Source: CAD feature listing. Evaluate the final solid. Frame: model axes, mm. Coordinates: 2 decimals unless noted, no trailing zeros. Order: outer loops, then holes, each group sorted by start corner. A loop starts at its lowest first (then second) coordinate and runs counter-clockwise, first axis right, second up.
Item 1: Section A-A on z = -14.5. Return the cut outline in (x, y).
Item 2: Section C-C on x = 3.35. State how many separate pieces and enclosed holes the cut face has, then the cut area to 3 significant figures.
Item 3: Ray query, line 1 (Z direction, x = 3.15, y = 330.2); line 2 (Z direction, x = 1.1, y = 429); line 3 (Y direction, x = 2, z = 17.5). Return the intervals inside material, ascending.
Item 4: Section B-B on y = 362. Return the cut outline in (x, z), then the cut area to 3 significant figures.
Autodesk Inventor part; units mm, degrees
ref_plane "YZ Plane" through (0, 0, 0) normal (1, 0, 0) x (0, 1, 0)
ref_plane "XZ Plane" through (0, 0, 0) normal (0, 1, 0) x (-1, 0, 0)
ref_plane "XY Plane" through (0, 0, 0) normal (0, 0, 1) x (1, 0, 0)
sketch "Sketch1" plane through (0, 0, 0) normal (1, 0, 0) x (0, 1, 0)
  line L0 (0, 50.8) -> (579.12, 50.8)
  line L1 (579.12, 50.8) -> (579.12, -50.8)
  line L2 (579.12, -50.8) -> (0, -50.8)
  line L3 (0, -50.8) -> (0, 50.8)
  point P0 (0, 0)
  point P1 (0, 0)
  dimension "d0" = 579.12
  dimension "d1" = 101.6
extrude "Extrusion1" add sketch "Sketch1" along normal blind 5.08
sketch "Sketch2" plane through (5.08, 0, 0) normal (1, 0, 0) x (0, 0, -1)
  line L0 (-50.8, 579.12) -> (-50.8, 0)
  line L1 (-50.8, 0) -> (50.8, 0)
  line L2 (50.8, 0) -> (50.8, 579.12)
  line L3 (50.8, 579.12) -> (-50.8, 579.12)
  line L4 (-25.4, 553.72) -> (-25.4, 25.4)
  line L5 (-25.4, 25.4) -> (25.4, 25.4)
  line L6 (25.4, 25.4) -> (25.4, 553.72)
  line L7 (25.4, 553.72) -> (-25.4, 553.72)
  point P0 (0, 0)
  dimension "d4" = 50.8
extrude "Extrusion2" cut sketch "Sketch2" against normal blind 5.08 contours L7 L6 L5 L4
sketch "Sketch3" plane through (5.08, 0, 0) normal (1, 0, 0) x (0, 0, -1)
  circle A0 centre (-40.64, 45.72) radius 2
  circle A1 centre (40.64, 5.08) radius 2
  circle A2 centre (-40.64, 5.08) radius 2
  circle A3 centre (40.64, 45.72) radius 2
  line L0 (-42.545, 0) -> (42.545, 0)
  line L1 (45.72, 3.175) -> (45.72, 62.865)
  line L2 (42.545, 66.04) -> (38.735, 66.04)
  line L3 (35.56, 62.865) -> (35.56, 10.16)
  line L4 (35.56, 10.16) -> (-35.56, 10.16)
  line L5 (-35.56, 10.16) -> (-35.56, 62.865)
  line L6 (-38.735, 66.04) -> (-42.545, 66.04)
  line L7 (-45.72, 62.865) -> (-45.72, 3.175)
  arc A4 (-45.72, 3.175) -> (-42.545, 0) centre (-42.545, 3.175) ccw
  arc A5 (42.545, 0) -> (45.72, 3.175) centre (42.545, 3.175) ccw
  arc A6 (45.72, 62.865) -> (42.545, 66.04) centre (42.545, 62.865) ccw
  arc A7 (38.735, 66.04) -> (35.56, 62.865) centre (38.735, 62.865) ccw
  arc A8 (-35.56, 62.865) -> (-38.735, 66.04) centre (-38.735, 62.865) ccw
  arc A9 (-42.545, 66.04) -> (-45.72, 62.865) centre (-42.545, 62.865) ccw
  point P0 (0, 0)
  point P1 (-40.64, 45.72)
  point P2 (40.64, 5.08)
  point P3 (40.64, 45.72)
  point P4 (-40.64, 86.36)
  point P5 (40.64, 86.36)
  point P6 (-40.64, 127)
  point P7 (40.64, 127)
  point P8 (-40.64, 167.64)
  point P9 (40.64, 167.64)
  point P10 (-40.64, 208.28)
  point P11 (40.64, 208.28)
  point P12 (-40.64, 248.92)
  point P13 (40.64, 248.92)
  point P14 (-40.64, 289.56)
  point P15 (40.64, 289.56)
  point P16 (-40.64, 330.2)
  point P17 (40.64, 330.2)
  point P18 (-40.64, 370.84)
  point P19 (40.64, 370.84)
  point P20 (-40.64, 411.48)
  point P21 (40.64, 411.48)
  point P22 (-40.64, 452.12)
  point P23 (40.64, 452.12)
  point P24 (-40.64, 492.76)
  point P25 (40.64, 492.76)
  point P26 (-40.64, 533.4)
  point P27 (40.64, 533.4)
  point P28 (-40.64, 574.04)
  point P29 (40.64, 574.04)
  dimension "d9" = 40.64
hole "Hole1" at (5.08, 5.08, 40.64) at (5.08, 45.72, 40.64) at (5.08, 5.08, -40.64) at (5.08, 45.72, -40.64) at (5.08, 86.36, 40.64) at (5.08, 86.36, -40.64) at (5.08, 127, 40.64) at (5.08, 127, -40.64) at (5.08, 167.64, 40.64) at (5.08, 167.64, -40.64) at (5.08, 208.28, 40.64) at (5.08, 208.28, -40.64) at (5.08, 248.92, 40.64) at (5.08, 248.92, -40.64) at (5.08, 289.56, 40.64) at (5.08, 289.56, -40.64) at (5.08, 330.2, 40.64) at (5.08, 330.2, -40.64) at (5.08, 370.84, 40.64) at (5.08, 370.84, -40.64) at (5.08, 411.48, 40.64) at (5.08, 411.48, -40.64) at (5.08, 452.12, 40.64) at (5.08, 452.12, -40.64) at (5.08, 492.76, 40.64) at (5.08, 492.76, -40.64) at (5.08, 533.4, 40.64) at (5.08, 533.4, -40.64) at (5.08, 574.04, 40.64) at (5.08, 574.04, -40.64) direction (-1, 0, 0) diameter 4 end through all
properties part number "Arm" material "Wood (Birch)"
Answer list:
1. outline: (0, 0) - (5.08, 0) - (5.08, 25.4) - (0, 25.4) - close; (0, 553.72) - (5.08, 553.72) - (5.08, 579.12) - (0, 579.12) - close
2. separate pieces: 1
2. enclosed holes: 31
2. area: 31,600 mm2
3. line 1: z = -50.8 to -42.64, -38.64 to -25.4, 25.4 to 38.64, 42.64 to 50.8
3. line 2: z = -50.8 to -25.4, 25.4 to 50.8
3. line 3: y = 0 to 25.4, 553.72 to 579.12
4. outline: (0, -50.8) - (5.08, -50.8) - (5.08, -25.4) - (0, -25.4) - close; (0, 25.4) - (5.08, 25.4) - (5.08, 50.8) - (0, 50.8) - close
4. area: 258 mm2
